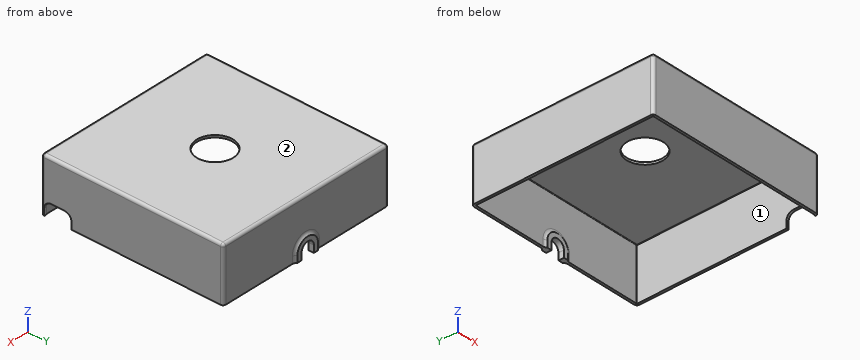
```python
from build123d import *

# Parameters (mm, degrees)
F0_W          = 200
F0_H          = 200
F0_R          = 20
F1_DEPTH      = 60
F2_R          = 3
F3_T          = -2.5
F4_DEPTH      = 60
F6_DEPTH      = 25
F8_DEPTH      = 25
F9_DEPTH      = 2
F9_DEPTH_BACK = 4
F10_T1_DEPTH  = 7.5
F10_T4_ANGLE  = 180
F10_T6_ANGLE  = 180


# Not quite as in the source:
# - a fillet or chamfer that OpenCascade refuses, or shapes differently, is made with other operations: its cross-section is extruded or revolved along the edge and cut away or added


with BuildPart() as f1:
    # F0 (on Top) → F1 (new body)
    with BuildSketch(Plane.XY):
        with Locations((100, -100)):
            Rectangle(F0_W, F0_H)
        with Locations((100, -100)):
            Circle(F0_R, mode=Mode.SUBTRACT)
        with Locations((100, -100)):
            Circle(F0_R)
    extrude(amount=F1_DEPTH)

    # F2
    f2_edges = [f1.edges().sort_by_distance(p)[0] for p in [
        (100, 0, 60),
        (200, -100, 60),
        (100, -200, 60),
        (0, -100, 60),
        (0, 0, 30),
        (0, -200, 30),
        (200, -200, 30),
        (200, 0, 30),
    ]]
    fillet(f2_edges, radius=F2_R)

    # F3
    f3_openings = [f1.faces().sort_by_distance(p)[0] for p in [
        (100, -100, 0),
    ]]
    offset(amount=F3_T, openings=f3_openings)

    # F0 (on Top) → F4 (cut, through all)
    with BuildSketch(Plane.XY):
        with Locations((100, -100)):
            Circle(F0_R)
    extrude(amount=F4_DEPTH, mode=Mode.SUBTRACT)

    # F5 (on face) → F6 (cut)
    with BuildSketch(Plane.YZ.offset(200)):
        with BuildLine():
            Line((-197, 7.5), (-197, 0))
            Line((-197, 0), (-167, 0))
            Line((-167, 0), (-167, 7.5))
            ThreePointArc((-167, 7.5), (-169.1966991411, 12.8033008589), (-174.5, 15))
            Line((-174.5, 15), (-189.5, 15))
            ThreePointArc((-189.5, 15), (-194.8033008589, 12.8033008589), (-197, 7.5))
        make_face()
    extrude(amount=-F6_DEPTH, mode=Mode.SUBTRACT)

    # F7 (on face) → F8 (cut)
    with BuildSketch(Plane(origin=(0, 0, 0), x_dir=(-1, 0, 0), z_dir=(0, 1, 0))):
        with BuildLine():
            Line((-92.5, 0), (-92.5, 7.5))
            ThreePointArc((-92.5, 7.5), (-100, 15), (-107.5, 7.5))
            Line((-107.5, 7.5), (-107.5, 0))
            Line((-107.5, 0), (-92.5, 0))
        make_face()
    extrude(amount=-F8_DEPTH, mode=Mode.SUBTRACT)

    # F7 (on face) → F9 (join, two sides)
    with BuildSketch(Plane(origin=(0, 0, 0), x_dir=(-1, 0, 0), z_dir=(0, 1, 0))) as f9_sk:
        with BuildLine():
            ThreePointArc((-107.5, 7.5), (-100, 15), (-92.5, 7.5))
            Line((-92.5, 7.5), (-92.5, 0))
            Line((-92.5, 0), (-87.5, 0))
            Line((-87.5, 0), (-87.5, 7.5))
            ThreePointArc((-87.5, 7.5), (-100, 20), (-112.5, 7.5))
            Line((-112.5, 7.5), (-112.5, 0))
            Line((-112.5, 0), (-107.5, 0))
            Line((-107.5, 0), (-107.5, 7.5))
        make_face()
    extrude(amount=F9_DEPTH)
    extrude(f9_sk.sketch, amount=-F9_DEPTH_BACK)

    # F10: fillet of radius 5 on 2 edges, made by hand

    # F10_s2 → F10_t1 (join)
    with BuildSketch(Plane.XY):
        with BuildLine():
            ThreePointArc((116.0707142143, -2.5), (114.1342225412, -2.8902277714), (112.5, -4))
            Line((112.5, -4), (112.5, -2.5))
            Line((112.5, -2.5), (116.0707142143, -2.5))
        make_face()
        with BuildLine():
            ThreePointArc((83.9292857857, -2.5), (85.8657774588, -2.8902277714), (87.5, -4))
            Line((87.5, -4), (87.5, -2.5))
            Line((87.5, -2.5), (83.9292857857, -2.5))
        make_face()
        with BuildLine():
            ThreePointArc((116.5, 0), (114.2639320225, 0.527864045), (112.5, 2))
            Line((112.5, 2), (112.5, 0))
            Line((112.5, 0), (116.5, 0))
        make_face()
        with BuildLine():
            ThreePointArc((83.5, 0), (85.7360679775, 0.527864045), (87.5, 2))
            Line((87.5, 2), (87.5, 0))
            Line((87.5, 0), (83.5, 0))
        make_face()
    extrude(amount=F10_T1_DEPTH)

    # F10_s3 → F10_t4 (revolve)
    with BuildSketch(Plane.XY.offset(7.5)):
        with BuildLine():
            ThreePointArc((116.5, 0), (114.2639320225, 0.527864045), (112.5, 2))
            Line((112.5, 2), (112.5, 0))
            Line((112.5, 0), (116.5, 0))
        make_face()
    revolve(axis=Axis((100, 0, 7.5), (0, -1, 0)), revolution_arc=F10_T4_ANGLE)

    # F10_s5 → F10_t6 (revolve)
    with BuildSketch(Plane.XY.offset(7.5)):
        with BuildLine():
            ThreePointArc((116.0707142143, -2.5), (114.1342225412, -2.8902277714), (112.5, -4))
            Line((112.5, -4), (112.5, -2.5))
            Line((112.5, -2.5), (116.0707142143, -2.5))
        make_face()
    revolve(axis=Axis((100, -2.5, 7.5), (0, -1, 0)), revolution_arc=F10_T6_ANGLE)


solid = f1.part
```
Verification items for the finished model (mm, model axes). Face numbers are marked on the shaded views. Round coordinates to 2 decimals unless told otherwise and drop trailing zeros. Write each loop counter-clockwise with the first axis right and the second up, starting at its lowest first coordinate (ties: lowest second). Pieces come first, ordered by that corner, then holes. Notation, with made-up numbers: (82, -11.75) -> (107, -11.75) arc R21 cw to (107, 2.25) -> close; hole circle Ø3 at (0, 25). An arc over 180 degrees is marked (long way). Write each question's results on one line, items separated by ' | '. Start each with the question number.
1. Material ranges on probe 1 along X at (y, z) = (-121, 38.5); probe 2 along Y at (x, z) = (163, 31); probe 3 along Z at (x, y) = (30.5, -70), recorded low to high. Write a range as from..to.
2. Draft check along Z on the marked faces 1 and 2. Enter one of: +Z half, -Z half, draft (parallel to the pull), parting line (faces both ways), or undercut.
3. Cross-section at B-B (x = 100). Enter the section's corners in (y, z), then the cut area to 3 significant figures.
4. Cross-section at C-C (z = 36). Enter the section's corners in (x, y).
5. Cross-section at A-A (y = -100). Enter the section's corners in (x, z), then the cut area to 3 significant figures.
6. Depth check by flat-ended pin: P1, Ø5, axis at x = 78.5, z = 31.5, coming from the +Y side; P2, Ø5, axis at x = 92.5, y = -131, coming from the -Z side; P3, Ø3, axis at x = 199, y = -184.5, coming from the -Z side. Enter the tip coordinate at first touch or a pass-through.
7. Cross-section at D-D (y = -184). Enter the section's corners in (x, z).
Solutions:
1) probe 1: x = 0..2.5, 197.5..200 | probe 2: y = -200..-197.5, -2.5..0 | probe 3: z = 57.5..60
2) face 1: draft | face 2: +Z half
3) outline: (-200, 0) -> (-197.5, 0) -> (-197.5, 57) arc R0.5 cw to (-197, 57.5) -> (-120, 57.5) -> (-120, 60) -> (-197, 60) arc R3 ccw to (-200, 57) -> close; (-80, 57.5) -> (-3, 57.5) arc R0.5 cw to (-2.5, 57) -> (-2.5, 23.57) arc R5 cw to (-4, 20) -> (-4, 15) -> (2, 15) -> (2, 20) arc R5 cw to (0, 24) -> (0, 57) arc R3 ccw to (-3, 60) -> (-80, 60) -> close | area: 668 mm2
4) outline: (0, -197) arc R3 ccw to (3, -200) -> (197, -200) arc R3 ccw to (200, -197) -> (200, -3) arc R3 ccw to (197, 0) -> (3, 0) arc R3 ccw to (0, -3) -> close; hole (2.5, -197) arc R0.5 ccw to (3, -197.5) -> (197, -197.5) arc R0.5 ccw to (197.5, -197) -> (197.5, -3) arc R0.5 ccw to (197, -2.5) -> (3, -2.5) arc R0.5 ccw to (2.5, -3) -> close
5) outline: (0, 0) -> (2.5, 0) -> (2.5, 57) arc R0.5 cw to (3, 57.5) -> (80, 57.5) -> (80, 60) -> (3, 60) arc R3 ccw to (0, 57) -> close; (120, 57.5) -> (197, 57.5) arc R0.5 cw to (197.5, 57) -> (197.5, 0) -> (200, 0) -> (200, 57) arc R3 ccw to (197, 60) -> (120, 60) -> close | area: 684 mm2
6) P1: stops at y = 0 | P2: stops at z = 57.5 | P3: stops at z = 15
7) outline: (0, 0) -> (2.5, 0) -> (2.5, 57) arc R0.5 cw to (3, 57.5) -> (197, 57.5) arc R0.5 cw to (197.5, 57) -> (197.5, 15) -> (200, 15) -> (200, 57) arc R3 ccw to (197, 60) -> (3, 60) arc R3 ccw to (0, 57) -> close
